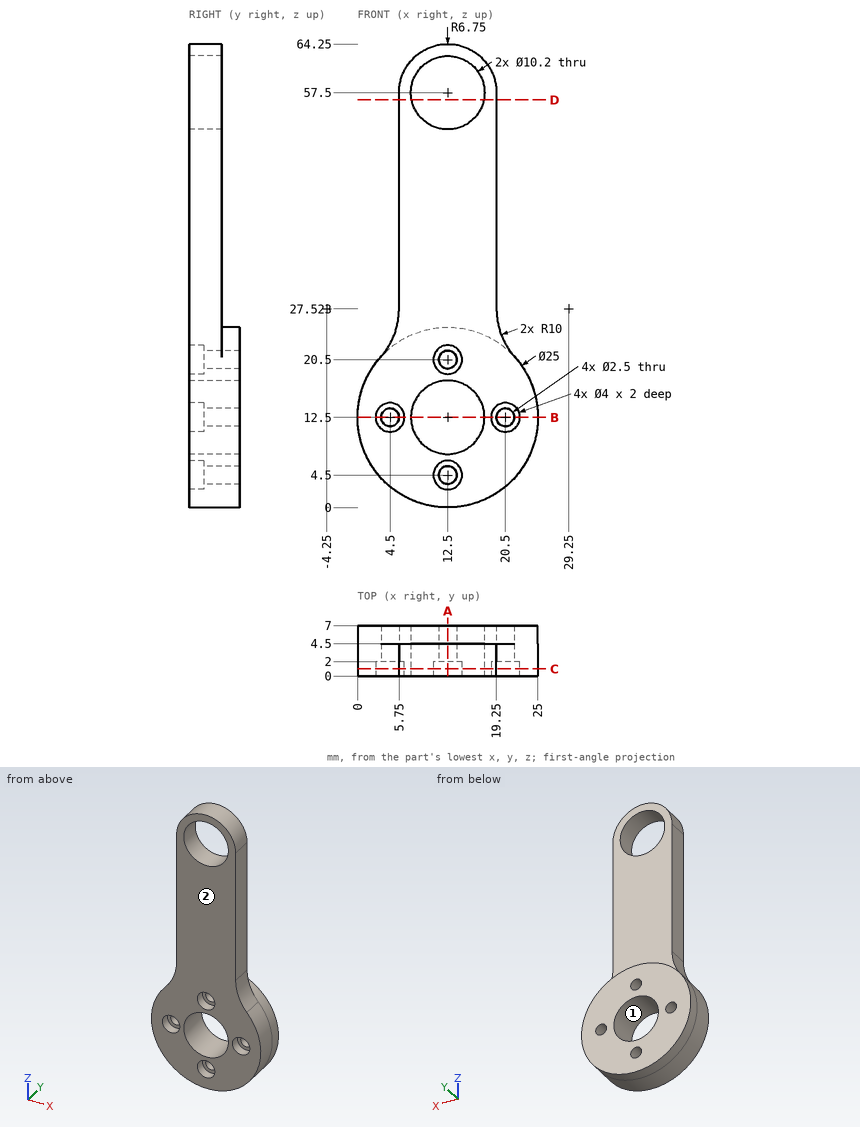
Could you check a few things on this drawing? It's one solid part, dimensions in mm from its lowest x, y, z. Round coordinates to 2 decimals unless told otherwise and drop trailing zeros. Loops run counter-clockwise (first coordinate to the right, second up) from the corner with the lowest first, then second, coordinate; pieces in that order, holes last. Notation, with made-up numbers: M -24,28 L -3,28 A31 cw -3,59 Z; hole C 34.5,-35 d10. An arc over 180 degrees is marked long. Write item = value, one per line. Start each with the question number.
(1) I need wall thicknesses on line 1 along Z through (x, y) = (12.5, 1.1); line 2 along Z through (x, y) = (12.5, 4.25); line 3 along X through (y, z) = (1.95, 57.5). Which ranges of each line are inside material? Lowest first, please.
(2) If we mould it in two halves opening along Z, with no side actions, what happens to the marked faces 1 and 2? For each: released by +Z, released by -Z, zero draft, split by the parting line, or undercut.
(3) I'm going to push flat-ended pins straight in: P1, Ø3, axis at x = 5.5, y = 3.5, coming from the -Z side (3 decimals); P2, Ø2, axis at y = 2.5, z = 43, coming from the +X side; P3, Ø5.5, axis at x = 11.5, z = 53.5, coming from the +Y side. Where does each tip first touch, or does it pass through?
(4) Suppose I cut it at D-D on z = 56.5. Write out the boundary of the cut face in (x, y), plus the area to 3 significant figures.
(5) Suppose I cut it at B-B on z = 12.5. Write out the boundary of the cut face in (x, y), plus the area to 3 significant figures.
(6) Suppose I cut it at C-C on y = 1. Write out the boundary of the cut face in (x, z).
(7) Suppose I cut it at A-A on x = 12.5. Give the number of separate pieces and of enclosed holes in the cut face, plus the area to 3 significant figures.
Answer block:
q1.line_1 = 0 to 2.5, 6.5 to 7.4, 17.6 to 18.5, 22.5 to 52.4, 62.6 to 64.25
q1.line_2 = 0 to 3.25, 5.75 to 7.4, 17.6 to 19.25, 21.75 to 52.4, 62.6 to 64.25
q1.line_3 = 5.75 to 7.4, 17.6 to 19.25
q2.face_1 = undercut
q2.face_2 = zero draft
q3.P1 = 1.275
q3.P2 = 19.25
q3.P3 = 4.5
q4.outline = M 5.75,0 L 7.5,0 L 7.5,4.5 L 5.75,4.5 Z; M 17.5,0 L 19.25,0 L 19.25,4.5 L 17.5,4.5 Z
q4.area = 15.7 mm²
q5.outline = M 0,0 L 2.5,0 L 2.5,2 L 3.25,2 L 3.25,7 L 0,7 Z; M 5.75,2 L 6.5,2 L 6.5,0 L 7.4,0 L 7.4,7 L 5.75,7 Z; M 17.6,0 L 18.5,0 L 18.5,2 L 19.25,2 L 19.25,7 L 17.6,7 Z; M 21.75,2 L 22.5,2 L 22.5,0 L 25,0 L 25,7 L 21.75,7 Z
q5.area = 62.6 mm²
q6.outline = M 3.19,20.85 A12.5 ccw long 21.81,20.85 A10 cw 19.25,27.52 L 19.25,57.5 A6.75 ccw 5.75,57.5 L 5.75,27.52 A10 cw Z; hole C 4.5,12.5 d4; hole C 12.5,12.5 d10.2; hole C 12.5,57.5 d10.2; hole C 12.5,4.5 d4; hole C 12.5,20.5 d4; hole C 20.5,12.5 d4
q7.separate_pieces = 5
q7.enclosed_holes = 0
q7.area = 193 mm²
